Input: part model. Units: mm. Frame: model coordinates. A direction names the side the tool comes from. Coordinates: 2 decimals unless noted, no trailing zeros. Order: outer loops, then holes, each group sorted by start corner. A loop starts at its lowest first (then second) coordinate and runs counter-clockwise, first axis right, second up. Notation, with made-up numbers: (-1, 23) - (55, 23) arc R29 ccw to (55, 55) - close; hole circle Ø5 at (23.25, -3). An arc over 180 degrees is marked (long way). Answer as CSV lines item,"result". Start each with the question number.
Item 1: Section D-D (z = -8.5). Output: boundary loops of the cut face in (x, y).
Item 2: Section B-B (x = -8). Output: boundary loops of the cut face in (y, z), and give its area (3 significant figures).
Item 3: First-contact query: pin 1 (1.5 mm diameter, centred on x = -8, z = -1, fed in from +Y); pin 2 (1 mm diameter, centred on x = 4.5, y = 21, fed in from +Z); pin 3 (2 mm diameter, centred on x = 7.5, z = -16.5, fed in from -Y). Flat tips, straight axial feed; report the tip coordinate or a pass-through.
Item 4: Draft query along Z for faces 3 (the cylindrical face through (8.496, 20.278, -4.047)), 4 (the flat face through (11.935, 19.389, 1.461)), 5 (the flat face through (0, 12.25, -2)). Return one class per face: +Z half, -Z half, draft (parallel to the pull), parting line (faces both ways), or undercut.
Item 5: Material intervals for line 1 along X through (y, z) = (18.75, -1.5); line 2 along Y through (x, z) = (11.25, 0); line 3 along X through (y, z) = (17.5, -2.5), sorted ascending.
Item 6: Section A-A (y = 15). Output: boundary loops of the cut face in (x, z) (3 decimals).
Item 7: Access query for faces 1 (the flat face through (-12.547, 20, -10)), 2 (the flat face through (-2, 17.25, -14)). Directions: +Z, -Z, +X, -X, +Y, -Y. A direction counts if a zero-diameter tool reaches every point of the face in a straight line with its end or side. Return the directions, or none.
Item 8: Section C-C (y = 21). Output: boundary loops of the cut face in (x, z), and give its area (3 significant figures).
from build123d import *
from OCP.BRepFilletAPI import BRepFilletAPI_MakeChamfer

# Parameters (mm, degrees)
SKETCH4_W                = 12.46
SKETCH4_H                = 17.25
BOSS_EXTRUDE3_DEPTH      = 6
BOSS_EXTRUDE6_DEPTH      = 7.3
BOSS_EXTRUDE6_DEPTH_BACK = 17.25
SKETCH8_R                = 12.546781182
SKETCH8_R_2              = 11.15
BOSS_EXTRUDE4_DEPTH      = 17.25
SKETCH6_R                = 2
CUT_EXTRUDE1_DEPTH       = 5
CHAMFER1_SIZE            = 0.5
CHAMFER1_SIZE_2          = 0.866025404
SKETCH10_W               = 12.46
SKETCH10_H               = 23.7
CUT_EXTRUDE3_DEPTH       = 17.25
CUT_EXTRUDE4_REACH       = 43.938
SKETCH11_W               = 5
SKETCH11_H               = 3
BOSS_EXTRUDE7_START      = -7.3
BOSS_EXTRUDE7_DEPTH      = 7.3
BOSS_EXTRUDE9_START      = 10
BOSS_EXTRUDE9_DEPTH      = 10
BOSS_EXTRUDE10_DEPTH     = 25.093562364
SKETCH18_W               = 21.5
SKETCH18_H               = 12.438292938
CUT_EXTRUDE5_DEPTH       = 2
CUT_EXTRUDE6_DEPTH       = 58.154608998
CUT_EXTRUDE6_DEPTH_BACK  = 58.154608998
SKETCH19_R               = 3.5
FILLET1_R                = 7
CUT_EXTRUDE7_DEPTH       = 55.97840444
CUT_EXTRUDE7_DEPTH_BACK  = 55.97840444
SKETCH20_W               = 25.093562364
SKETCH20_H               = 36.096781182
BOSS_EXTRUDE11_DEPTH     = 44.5
CUT_EXTRUDE8_DEPTH       = 40.401576339
CUT_EXTRUDE8_DEPTH_BACK  = 40.401576339
CUT_EXTRUDE9_DEPTH       = 40.401576339
SKETCH24_R               = 6.5
BOSS_EXTRUDE12_DEPTH     = 5
SKETCH25_R               = 6.075
BOSS_EXTRUDE13_DEPTH     = 5
FILLET2_R                = 1
BOSS_EXTRUDE14_DEPTH     = 2
CUT_EXTRUDE10_REACH      = 57.104
SKETCH27_R               = 0.75
CUT_EXTRUDE11_DEPTH      = 45.983908275
CUT_EXTRUDE11_DEPTH_BACK = 45.983908275
CUT_EXTRUDE12_DEPTH      = 30.927775026
CUT_EXTRUDE12_DEPTH_BACK = 30.927775026
SKETCH29_R               = 1.65
SKETCH30_R               = 2.25
BOSS_EXTRUDE15_DEPTH     = 6
FILLET3_R                = 1


with BuildPart() as part:
    # Sketch4 → Boss-Extrude3 (new body)
    with BuildSketch(Plane.XY):
        with Locations((0, -1.35)):
            Rectangle(SKETCH4_W, SKETCH4_H)
    extrude(amount=BOSS_EXTRUDE3_DEPTH)



with BuildPart() as body_2:
    # Sketch8 → Boss-Extrude6 (new, two sides: drawn at the far end of the back side and taken through both)
    with BuildSketch(Plane(origin=(0, -9.975, 0), x_dir=(-1, 0, 0), z_dir=(0, -1, 0)).offset(-BOSS_EXTRUDE6_DEPTH_BACK)):
        with Locations(Location((0, -23.55, 0), (0, 0, 90))):
            Circle(SKETCH8_R)
        with Locations(Location((0, -23.55, 0), (0, 0, 90))):
            Circle(SKETCH8_R_2, mode=Mode.SUBTRACT)
    extrude(amount=BOSS_EXTRUDE6_DEPTH + BOSS_EXTRUDE6_DEPTH_BACK)


with BuildPart() as part_1:
    add(part.part)

    add(body_2.part)  # Boss-Extrude4 merges body 2
    # Sketch5 → Boss-Extrude4 (add)
    with BuildSketch(Plane(origin=(0, 7.275, 0), x_dir=(1, 0, 0), z_dir=(0, 1, 0))):
        with BuildLine():
            Line((12.546781182, -23.55), (12.546781182, 0))
            Line((12.546781182, 0), (6.23, 0))
            Line((6.23, 0), (6.23, -29.7))
            Line((6.23, -29.7), (-6.23, -29.7))
            Line((-6.23, -29.7), (-6.23, 0))
            Line((-6.23, 0), (-12.546781182, 0))
            Line((-12.546781182, 0), (-12.546781182, -23.55))
            ThreePointArc((-12.546781182, -23.55), (0, -36.096781182), (12.546781182, -23.55))
        make_face()
    extrude(amount=-BOSS_EXTRUDE4_DEPTH)

    # Sketch6 → Cut-Extrude1 (cut)
    with BuildSketch(Plane(origin=(0, 7.275, 0), x_dir=(1, 0, 0), z_dir=(0, 1, 0))):
        with Locations(Location((0, -3.5, 0), (0, 0, 270))):
            Circle(SKETCH6_R)
        with Locations(Location((0, -32.2, 0), (0, 0, 270))):
            Circle(SKETCH6_R)
    extrude(amount=-CUT_EXTRUDE1_DEPTH, mode=Mode.SUBTRACT)

    # Chamfer1
    chamfer1_edges_1 = [part_1.edges().sort_by_distance(p)[0] for p in [
        (0, 7.275, 1.5),
    ]]
    chamfer1_side_1 = [part_1.faces().sort_by_distance(p)[0] for p in [
        (0, 7.275, 1.49),
    ]]
    chamfer1_edges_2 = [part_1.edges().sort_by_distance(p)[0] for p in [
        (0, 7.275, 30.2),
    ]]
    chamfer1_side_2 = [part_1.faces().sort_by_distance(p)[0] for p in [
        (0, 7.275, 30.19),
    ]]
    chamfer1 = BRepFilletAPI_MakeChamfer(part_1.part.solid().wrapped)
    for e in chamfer1_edges_1:
        chamfer1.Add(CHAMFER1_SIZE - 0.0001, CHAMFER1_SIZE_2 - 0.0001, e.wrapped, chamfer1_side_1[0].wrapped)
    for e in chamfer1_edges_2:
        chamfer1.Add(CHAMFER1_SIZE - 0.0001, CHAMFER1_SIZE_2 - 0.0001, e.wrapped, chamfer1_side_2[0].wrapped)
    add(Compound.cast(chamfer1.Shape()), mode=Mode.REPLACE)  # a hair under: the kernel refuses the full size

    # Sketch10 → Cut-Extrude3 (cut)
    with BuildSketch(Plane(origin=(0, 7.275, 0), x_dir=(1, 0, 0), z_dir=(0, 1, 0))):
        with Locations((0, -17.85)):
            Rectangle(SKETCH10_W, SKETCH10_H)
    extrude(amount=-CUT_EXTRUDE3_DEPTH, mode=Mode.SUBTRACT)

    # Sketch11 → Cut-Extrude4 (cut, up to next)
    with BuildSketch(Plane.XY.offset(36.096781182), mode=Mode.PRIVATE) as cut_extrude4_sk1:
        with Locations((0, -8.475)):
            Rectangle(SKETCH11_W, SKETCH11_H)
    cut_extrude4_tool1 = extrude(cut_extrude4_sk1.sketch, amount=-CUT_EXTRUDE4_REACH, mode=Mode.PRIVATE) & part_1.part
    add(cut_extrude4_tool1.solids().sort_by_distance((0, -8.475, 36.096781))[0], mode=Mode.SUBTRACT)

    # Sketch13 → Boss-Extrude7 (add)
    with BuildSketch(Plane.XZ.offset(17.275).offset(BOSS_EXTRUDE7_START)):
        with BuildLine():
            Line((-12.546781182, 23.55), (-12.546781182, 0))
            Line((-12.546781182, 0), (12.546781182, 0))
            Line((12.546781182, 0), (12.546781182, 23.55))
            ThreePointArc((12.546781182, 23.55), (0, 11.003218818), (-12.546781182, 23.55))
        make_face()
    extrude(amount=BOSS_EXTRUDE7_DEPTH)

    # Sketch15 → Boss-Extrude9 (add)
    with BuildSketch(Plane(origin=(0, 7.275, 0), x_dir=(1, 0, 0), z_dir=(0, 1, 0)).offset(BOSS_EXTRUDE9_START)):
        with BuildLine():
            Line((-12.546781182, 0), (12.546781182, 0))
            Line((12.546781182, 0), (12.546781182, -23.55))
            ThreePointArc((12.546781182, -23.55), (0, -36.096781182), (-12.546781182, -23.55))
            Line((-12.546781182, -23.55), (-12.546781182, 0))
        make_face()
        with BuildLine():
            Line((-6.23, -0.8), (6.23, -0.8))
            Line((6.23, -0.8), (6.23, -33.5))
            ThreePointArc((6.23, -33.5), (5.937106781, -34.207106781), (5.23, -34.5))
            Line((5.23, -34.5), (-5.23, -34.5))
            ThreePointArc((-5.23, -34.5), (-5.937106781, -34.207106781), (-6.23, -33.5))
            Line((-6.23, -33.5), (-6.23, -0.8))
        make_face(mode=Mode.SUBTRACT)
    extrude(amount=-BOSS_EXTRUDE9_DEPTH)

    # Sketch17 → Boss-Extrude10 (add)
    with BuildSketch(Plane(origin=(-12.546781182, 4.728218818, 0), x_dir=(0, -1, 0), z_dir=(1, 0, 0))):
        Polygon((26.978218818, 26.5), (26.978218818, 0), (-17.521781182, 0), (-17.521781182, 26.5), (-13.521781182, 26.5), (-13.521781182, 5), (22.978218818, 5), (22.978218818, 26.5), align=None)
    extrude(amount=BOSS_EXTRUDE10_DEPTH)

    # Sketch18 → Cut-Extrude5 (cut)
    with BuildSketch(Plane.ZX.offset(-18.25)):
        with Locations((-15.75, 0)):
            Rectangle(SKETCH18_W, SKETCH18_H)
    extrude(amount=-CUT_EXTRUDE5_DEPTH, mode=Mode.SUBTRACT)

    # Sketch19 → Cut-Extrude6 (cut, two sides: drawn at the far end of the back side and taken through both)
    with BuildSketch(Plane.ZX.offset(-20.25).offset(-CUT_EXTRUDE6_DEPTH_BACK)):
        with Locations((-20, 0)):
            Circle(SKETCH19_R)
    extrude(amount=CUT_EXTRUDE6_DEPTH + CUT_EXTRUDE6_DEPTH_BACK, mode=Mode.SUBTRACT)

    # Fillet1
    fillet1_edges = [part_1.edges().sort_by_distance(p)[0] for p in [
        (12.546781182, -20.25, -26.5),
        (-12.546781182, -20.25, -26.5),
        (-12.546781182, 20.25, -26.5),
        (12.546781182, 20.25, -26.5),
    ]]
    fillet(fillet1_edges, radius=FILLET1_R)

    # Sketch20 → Cut-Extrude7 (cut, two sides: drawn at the far end of the back side and taken through both)
    with BuildSketch(Plane(origin=(0, 17.275, 0), x_dir=(1, 0, 0), z_dir=(0, 1, 0)).offset(-CUT_EXTRUDE7_DEPTH_BACK)):
        with Locations((0, -18.048390591)):
            Rectangle(SKETCH20_W, SKETCH20_H)
    extrude(amount=CUT_EXTRUDE7_DEPTH + CUT_EXTRUDE7_DEPTH_BACK, mode=Mode.SUBTRACT)

    # Sketch21 → Boss-Extrude11 (add)
    with BuildSketch(Plane(origin=(0, 22.25, 0), x_dir=(1, 0, 0), z_dir=(0, 1, 0))):
        Polygon((12.546781182, 0), (-0.025415104, -30), (-12.546781182, 0), align=None)
    extrude(amount=-BOSS_EXTRUDE11_DEPTH)

    # Sketch22 → Cut-Extrude8 (cut, two sides: drawn at the far end of the back side and taken through both)
    with BuildSketch(Plane(origin=(0, 0, 0), x_dir=(0, 0, -1), z_dir=(1, 0, 0)).offset(-CUT_EXTRUDE8_DEPTH_BACK)):
        Polygon((0, 22.25), (-30, 0.01), (-30, 22.25), align=None)
        Polygon((0, -22.25), (-30, -22.25), (-30, -0.01), align=None)
    extrude(amount=CUT_EXTRUDE8_DEPTH + CUT_EXTRUDE8_DEPTH_BACK, mode=Mode.SUBTRACT)

    # Sketch23 → Cut-Extrude9 (cut, through all)
    with BuildSketch(Plane(origin=(0, 0, 0), x_dir=(-1, 0, 0), z_dir=(0, 0, -1))):
        Polygon((12.546781182, 18.25), (0, 0), (12.546781182, -22.25), align=None)
    extrude(amount=-CUT_EXTRUDE9_DEPTH, mode=Mode.SUBTRACT)

    # Sketch24 → Boss-Extrude12 (add)
    with BuildSketch(Plane(origin=(0, 22.25, 0), x_dir=(1, 0, 0), z_dir=(0, 1, 0))):
        with Locations(Location((0, 20, 0), (0, 0, 270))):
            Circle(SKETCH24_R)
    extrude(amount=-BOSS_EXTRUDE12_DEPTH)

    # Sketch25 → Boss-Extrude13 (add)
    with BuildSketch(Plane.XZ.offset(-17.25)):
        with Locations(Location((0, -20, 0), (0, 0, 270))):
            Circle(SKETCH25_R)
    extrude(amount=BOSS_EXTRUDE13_DEPTH)

    # Fillet2
    fillet2_edges = [part_1.edges().sort_by_distance(p)[0] for p in [
        (0, 12.25, -13.925),
    ]]
    fillet(fillet2_edges, radius=FILLET2_R)

    # Sketch26 → Boss-Extrude14 (add)
    with BuildSketch(Plane(origin=(0, -20.25, 0), x_dir=(1, 0, 0), z_dir=(0, 1, 0))):
        Polygon((-6.219146469, 5), (-2.5, 5), (-3.1585, 20), (-3.44385, 26.5), (-6.219146469, 26.5), align=None)
        Polygon((3.1585, 20), (3.44385, 26.5), (6.219146469, 26.5), (6.219146469, 5), (2.5, 5), align=None)
    extrude(amount=BOSS_EXTRUDE14_DEPTH)

    # Sketch27 → Cut-Extrude10 (cut, up to next)
    with BuildSketch(Plane.XZ.offset(22.25), mode=Mode.PRIVATE) as cut_extrude10_sk1:
        with Locations(Location((0, -10, 0), (0, 0, 270))):
            Circle(SKETCH27_R)
    cut_extrude10_tool1 = extrude(cut_extrude10_sk1.sketch, amount=-CUT_EXTRUDE10_REACH, mode=Mode.PRIVATE) & part_1.part
    # Sketch27 → Cut-Extrude10 (cut, up to next)
    with BuildSketch(Plane.XZ.offset(22.25), mode=Mode.PRIVATE) as cut_extrude10_sk2:
        with Locations(Location((0, -7.5, 0), (0, 0, 270))):
            Circle(SKETCH27_R)
    cut_extrude10_tool2 = extrude(cut_extrude10_sk2.sketch, amount=-CUT_EXTRUDE10_REACH, mode=Mode.PRIVATE) & part_1.part
    # Sketch27 → Cut-Extrude10 (cut, up to next)
    with BuildSketch(Plane.XZ.offset(22.25), mode=Mode.PRIVATE) as cut_extrude10_sk3:
        with Locations(Location((0, -12.5, 0), (0, 0, 270))):
            Circle(SKETCH27_R)
    cut_extrude10_tool3 = extrude(cut_extrude10_sk3.sketch, amount=-CUT_EXTRUDE10_REACH, mode=Mode.PRIVATE) & part_1.part
    add(cut_extrude10_tool1.solids().sort_by_distance((0, -22.25, -10))[0], mode=Mode.SUBTRACT)
    add(cut_extrude10_tool2.solids().sort_by_distance((0, -22.25, -7.5))[0], mode=Mode.SUBTRACT)
    add(cut_extrude10_tool3.solids().sort_by_distance((0, -22.25, -12.5))[0], mode=Mode.SUBTRACT)

    # Sketch28 → Cut-Extrude11 (cut, two sides: drawn at the far end of the back side and taken through both)
    with BuildSketch(Plane(origin=(12.546781182, 0, 0), x_dir=(0, 0, -1), z_dir=(1, 0, 0)).offset(-CUT_EXTRUDE11_DEPTH_BACK)):
        Polygon((5, 18.25), (-35.232883585, 18.25), (-35.232883585, -25.616523732), (31.598677018, -25.616523732), (31.598677018, 10.892065209), (5, 10.892065209), align=None)
    extrude(amount=CUT_EXTRUDE11_DEPTH + CUT_EXTRUDE11_DEPTH_BACK, mode=Mode.SUBTRACT)

    # Sketch29 → Cut-Extrude12 (cut, two sides: drawn at the far end of the back side and taken through both)
    with BuildSketch(Plane.XZ.offset(-18.25).offset(-CUT_EXTRUDE12_DEPTH_BACK)):
        with Locations(Location((-8, -2.473316547, 0), (0, 0, 270))):
            Circle(SKETCH29_R)
        with Locations(Location((8, -2.473316547, 0), (0, 0, 270))):
            Circle(SKETCH29_R)
    extrude(amount=CUT_EXTRUDE12_DEPTH + CUT_EXTRUDE12_DEPTH_BACK, mode=Mode.SUBTRACT)

    # Sketch30 → Boss-Extrude15 (add)
    with BuildSketch(Plane.XZ.offset(-18.25)):
        with Locations(Location((0, -2.473316547, 0), (0, 0, 90))):
            Circle(SKETCH30_R)
    extrude(amount=BOSS_EXTRUDE15_DEPTH)

    # Fillet3
    fillet3_edges = [part_1.edges().sort_by_distance(p)[0] for p in [
        (0, 12.25, -4.723316547),
    ]]
    fillet(fillet3_edges, radius=FILLET3_R)


solid = part_1.part
Determined:
1,outline,"(-12.55, 18.25) - (12.55, 18.25) - (12.55, 22.25) - (-12.55, 22.25) - close"
2,outline,"(18.25, -26.06) - (22.25, -26.06) - (22.25, -4.12) - (18.25, -4.12) - close; (18.25, -0.82) - (22.25, -0.82) - (22.25, 0) - (18.25, 5.4) - close"
2,area,"102 mm^2"
3,pin 1,"stops at y = 22.25"
3,pin 2,"stops at z = 2.36"
3,pin 3,"stops at y = 18.25"
4,face 3,"undercut"
4,face 4,"+Z half"
4,face 5,"draft"
5,line 1,"x = -12.55 to -9.33, -6.67 to 6.67, 9.33 to 12.55"
5,line 2,"y = 18.25 to 22.25"
5,line 3,"x = -2.25 to 2.25"
6,outline,"circle Ø12.15 at (0, -20); circle Ø4.5 at (0, -2.473)"
7,face 1,"+Z, -Z, -X, +Y, -Y"
7,face 2,"-Y"
8,outline,"(-12.55, -19.5) arc R7 ccw to (-5.55, -26.5) - (5.55, -26.5) arc R7 ccw to (12.55, -19.5) - (12.55, 0) - (11.84, 1.69) - (-11.84, 1.69) - (-12.55, 0) - close; hole circle Ø3.3 at (-8, -2.47); hole circle Ø3.3 at (8, -2.47)"
8,area,"668 mm^2"
